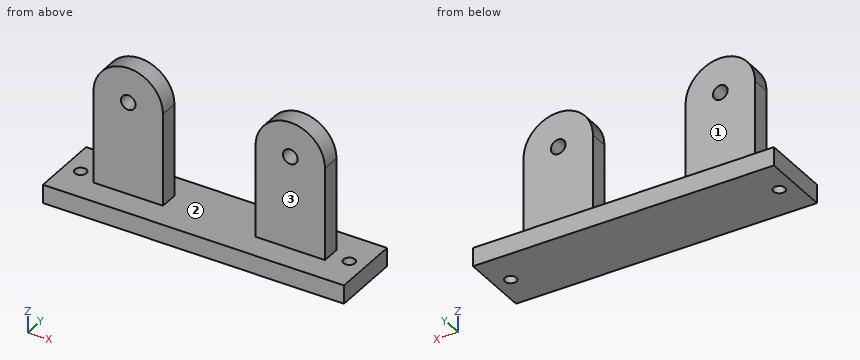
Autodesk Fusion 360 part; units mm, degrees
sketch "草图1" plane through (0, 0, 0) normal (0, 0, 1) x (1, 0, 0)
  line L0 (-65, 15) -> (65, 15)
  line L1 (65, 15) -> (65, -15)
  line L2 (65, -15) -> (-65, -15)
  line L3 (-65, -15) -> (-65, 15)
  line L4 (1.75, 0) -> (22.5, 0)
  line L5 (0, 1.75) -> (0, 22.5)
  circle A0 centre (58, 0) radius 2.5
  circle A1 centre (-58, 0) radius 2.5
  dimension "d1" = 130
  dimension "d2" = 30
  dimension "d16" = 5
  dimension "d17" = 58
  dimension "d18" = 5
extrude "拉伸1" add sketch "草图1" against normal blind 8
ref_plane "工作平面1" through (0, 4, 0) normal (0, 1, 0) x (0, 0, 1)
sketch "草图2" plane through (0, 4, 0) normal (0, 1, 0) x (1, 0, 0)
  line L0 (50, 0) -> (20, 0)
  line L1 (20, 0) -> (20, -40)
  line L2 (20, -40) -> (50, -40)
  line L3 (50, -40) -> (50, 0)
  circle A0 centre (35, -40) radius 15
  circle A1 centre (35, -40) radius 3.175
  dimension "d6" = 30
  dimension "d7" = 40
  dimension "d8" = 20
  dimension "d9" = 6.35
  dimension "d14" = 35
  dimension "d15" = 35
extrude "拉伸2" add sketch "草图2" against normal blind 8 contours L0 L1 L3 A0 | L2 A0 A1 | L2 A0 A1
mirror "镜像1" about plane through (0, 0, 0) normal (1, 0, 0) of bodies 1 merged
equation "d18 = d16"
Verification items for the finished model (mm, model axes). Face numbers are marked on the shaded views. A direction names the side the tool comes from. Coordinates: 2 decimals unless noted, no trailing zeros. Write each loop counter-clockwise with the first axis right and the second up, starting at its lowest first coordinate (ties: lowest second). Pieces come first, ordered by that corner, then holes. Notation, with made-up numbers: (68.25, -31) -> (87.25, -31) arc R35 ccw to (87.25, 1) -> close; hole circle Ø2 at (-6.75, -40). An arc over 180 degrees is marked (long way). One line per item, written item: value. Start each with the question number.
Q1. Go/stop test with flat-tipped pins: P1, Ø2, axis at x = -7.5, y = -6.5, coming from the +Z side; P2, Ø15, axis at x = -33, z = 23.5, coming from the -Y side; P3, Ø15, axis at x = 29.5, z = 19, coming from the +Y side. Record where each tip stops, or that it passes through.
Q2. Access from +Z, -Z, +X, -X, +Y, -Y to the whole of each face (thin tool, end or side, straight path). Record for the marked faces 1, 2 and 3.
Q3. Thickness scan on L1, parallel to X at y = 0, z = -4.25; L2, parallel to Y at x = 58, z = -4.5; L3, parallel to X at y = -1.25, z = 40 (3 decimals). Record the ranges inside material, lowest first. Write a range as from..to.
Q4. Cross-section at B-B on x = 35. Enter the section's corners in (y, z) (3 decimals).
Q5. Cross-section at C-C on z = 28. Enter the section's corners in (x, y).
Q6. Cross-section at A-A on y = 0. Enter the section's corners in (x, z) (3 decimals).
Q7. Cross-section at D-D on x = -24.5. Enter the section's corners in (y, z).
Checked values:
1. P1: stops at z = 0
1. P2: stops at y = -4
1. P3: stops at y = 4
2. face 1: +Z, +X, -X, +Y
2. face 2: +Z
2. face 3: +Z, +X, -X, -Y
3. L1: x = -65..-60.5, -55.5..55.5, 60.5..65
3. L2: y = -15..-2.5, 2.5..15
3. L3: x = -50..-38.175, -31.825..-20, 20..31.825, 38.175..50
4. outline: (-15, -8) -> (15, -8) -> (15, 0) -> (4, 0) -> (4, 36.825) -> (-4, 36.825) -> (-4, 0) -> (-15, 0) -> close; (-4, 43.175) -> (4, 43.175) -> (4, 55) -> (-4, 55) -> close
5. outline: (-50, -4) -> (-20, -4) -> (-20, 4) -> (-50, 4) -> close; (20, -4) -> (50, -4) -> (50, 4) -> (20, 4) -> close
6. outline: (-65, -8) -> (-60.5, -8) -> (-60.5, 0) -> (-65, 0) -> close; (-55.5, -8) -> (55.5, -8) -> (55.5, 0) -> (50, 0) -> (50, 40) arc R15 ccw to (20, 40) -> (20, 0) -> (-20, 0) -> (-20, 40) arc R15 ccw to (-50, 40) -> (-50, 0) -> (-55.5, 0) -> close; (60.5, -8) -> (65, -8) -> (65, 0) -> (60.5, 0) -> close; hole circle Ø6.35 at (-35, 40); hole circle Ø6.35 at (35, 40)
7. outline: (-15, -8) -> (15, -8) -> (15, 0) -> (4, 0) -> (4, 50.71) -> (-4, 50.71) -> (-4, 0) -> (-15, 0) -> close
